Part model, mm, in its own coordinate system. Give positions to 0.01 mm unless a question says otherwise; leave off trailing zeros. Write each loop counter-clockwise with the first axis right and the second up, starting at its lowest first coordinate (ties: lowest second). Pieces come first, ordered by that corner, then holes.
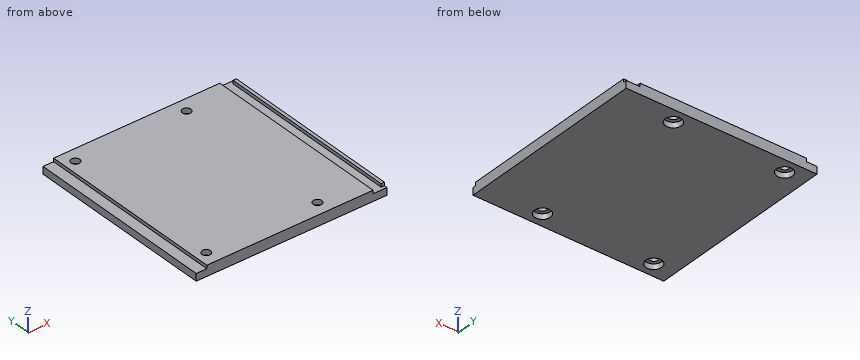
```python
from build123d import *

# Parameters (mm, degrees)
F0_W           = 72
F0_H           = 72
F1_DEPTH       = 2.75
F2_W           = 62.75
F2_H           = 72
F2_W_2         = 1.25
F3_DEPTH       = 1.25
F5_D           = 3.25
F5_DEPTH       = 8
F5_CBORE_D     = 6
F5_CBORE_DEPTH = 2
F6_W           = 1.25
F6_H           = 1.25
F7_DEPTH       = 1.25


with BuildPart() as f1:
    # F0 (on Top) → F1 (new body)
    with BuildSketch(Plane.XY):
        Rectangle(F0_W, F0_H)
    extrude(amount=F1_DEPTH)

    # F2 (on face) → F3 (join)
    with BuildSketch(Plane.XY.offset(2.75)):
        with Locations((-0.625, 0)):
            Rectangle(F2_W, F2_H)
        with Locations((35.375, 0)):
            Rectangle(F2_W_2, F2_H)
    extrude(amount=F3_DEPTH)

    # F5
    with Locations(Plane(origin=(0, 0, 0), x_dir=(1, 0, 0), z_dir=(0, 0, -1))):
        with Locations((-28, -30.75), (14, -30.75), (-28, 30.75), (14, 30.75)):
            CounterBoreHole(F5_D / 2, F5_CBORE_D / 2, F5_CBORE_DEPTH, depth=F5_DEPTH)

    # F6 (on face) → F7 (cut)
    with BuildSketch(Plane.XY.offset(4)):
        with Locations((35.375, 35.375)):
            Rectangle(F6_W, F6_H)
        with Locations((35.375, -35.375)):
            Rectangle(F6_W, F6_H)
    extrude(amount=-F7_DEPTH, mode=Mode.SUBTRACT)


solid = f1.part
```
1) Saw through at B-B, the plane x = 14. Write the cut outline in (y, z) (3 decimals), then the cut area to 3 significant figures.
Answers follow:
outline: (-36, 0) - (-33.75, 0) - (-33.75, 2) - (-32.375, 2) - (-32.375, 4) - (-36, 4) - close; (-29.125, 2) - (-27.75, 2) - (-27.75, 0) - (27.75, 0) - (27.75, 2) - (29.125, 2) - (29.125, 4) - (-29.125, 4) - close; (32.375, 2) - (33.75, 2) - (33.75, 0) - (36, 0) - (36, 4) - (32.375, 4) - close
area: 251 mm2
2) Saw through at C-C, the plane y = 9. Write the cut outline in (x, z), then the cut area to 3 significant figures.
Answers follow:
outline: (-36, 0) - (36, 0) - (36, 4) - (34.75, 4) - (34.75, 2.75) - (30.75, 2.75) - (30.75, 4) - (-32, 4) - (-32, 2.75) - (-36, 2.75) - close
area: 278 mm2
3) Saw through at A-A, the plane y = 30.75. Write the cut outline in (x, z) (3 decimals), then the cut area to 3 significant figures.
Answers follow:
outline: (-36, 0) - (-31, 0) - (-31, 2) - (-29.625, 2) - (-29.625, 4) - (-32, 4) - (-32, 2.75) - (-36, 2.75) - close; (-26.375, 2) - (-25, 2) - (-25, 0) - (11, 0) - (11, 2) - (12.375, 2) - (12.375, 4) - (-26.375, 4) - close; (15.625, 2) - (17, 2) - (17, 0) - (36, 0) - (36, 4) - (34.75, 4) - (34.75, 2.75) - (30.75, 2.75) - (30.75, 4) - (15.625, 4) - close
area: 241 mm2
4) Wall check: L1, parallel to Y at x = -28, z = 2.5 (3 decimals); L2, parallel to Y at x = -28, z = 1.25; L3, parallel to X at y = -30.75, z = 3.6 (3 decimals). Give the ranges that are in metal, low to high.
Answers follow:
L1: y = -36 to -32.375, -29.125 to 29.125, 32.375 to 36
L2: y = -36 to -33.75, -27.75 to 27.75, 33.75 to 36
L3: x = -32 to -29.625, -26.375 to 12.375, 15.625 to 30.75, 34.75 to 36
5) Pin check, flat tips, straight feed: pin 1 Ø3 at (x, y) = (-28, 30) entering from -Z; pin 2 Ø4 at (x, y) = (14, -30.75) entering from +Z; pin 3 Ø0.6 at (x, z) = (35, 3.5) entering from -Y; pin 4 Ø1.2 at (x, y) = (-34, -1.5) entering from +Z. Stop position of each tip, or through.
Answers follow:
pin 1: stops at z = 2
pin 2: stops at z = 4
pin 3: stops at y = -34.75
pin 4: stops at z = 2.75
